Read the model definition and answer for the solid it produces. Units are mm, in the model's axes. A direction names the side the tool comes from. Coordinates: 2 decimals unless noted, no trailing zeros. Order: outer loops, then holes, each group sorted by start corner. A loop starts at its lowest first (then second) coordinate and runs counter-clockwise, first axis right, second up. Notation, with made-up numbers: M 15.5,25.25 L 57.5,25.25 A19 ccw 57.5,49.25 Z; hole C 14,-26 d8. An arc over 180 degrees is marked long. Write each question's results on one line, items separated by ' | '.
```python
from build123d import *

# Parameters (mm, degrees)
SKETCH_1_W           = 17.78
SKETCH_1_H           = 6.35
EXTRUDE_1_DEPTH      = 5.08
SKETCH_2_W           = 16.78
SKETCH_2_H           = 5.35
CUT_EXTRUDE_1_DEPTH  = 4.08
SKETCH_3_W           = 2
SKETCH_3_H           = 4.08
CUT_EXTRUDE_2_DEPTH  = 1
EXTRUDE_2_DEPTH      = 2
EXTRUDE_2_DEPTH_BACK = 3.58
SKETCH_4_W           = 0.75
SKETCH_4_H           = 0.75


with BuildPart() as part:
    # 草图1 → 拉伸1 (new body)
    with BuildSketch(Plane(origin=(0, 0, 0), x_dir=(1, 0, 0), z_dir=(0, 1, 0))):
        Rectangle(SKETCH_1_W, SKETCH_1_H)
    extrude(amount=EXTRUDE_1_DEPTH)

    # 草图2 → 切除-拉伸1 (cut)
    with BuildSketch(Plane(origin=(0, 5.08, 0), x_dir=(-1, 0, 0), z_dir=(0, 1, 0))):
        Rectangle(SKETCH_2_W, SKETCH_2_H)
    extrude(amount=-CUT_EXTRUDE_1_DEPTH, mode=Mode.SUBTRACT)

    # 草图3 → 切除-拉伸2 (cut)
    with BuildSketch(Plane.XY.offset(3.175)):
        with Locations((0, 3.04)):
            Rectangle(SKETCH_3_W, SKETCH_3_H)
    extrude(amount=-CUT_EXTRUDE_2_DEPTH, mode=Mode.SUBTRACT)

    # 草图4 → 拉伸2 (add, two sides: drawn at the far end of the back side and taken through both)
    with BuildSketch(Plane.XZ.offset(-EXTRUDE_2_DEPTH_BACK)):
        with Locations((-1.27, 0.635)):
            Rectangle(SKETCH_4_W, SKETCH_4_H)
        with Locations((1.27, 0.635)):
            Rectangle(SKETCH_4_W, SKETCH_4_H)
        with Locations((3.81, 0.635)):
            Rectangle(SKETCH_4_W, SKETCH_4_H)
        with Locations((6.35, 0.635)):
            Rectangle(SKETCH_4_W, SKETCH_4_H)
        with Locations((-3.81, 0.635)):
            Rectangle(SKETCH_4_W, SKETCH_4_H)
        with Locations((-6.35, 0.635)):
            Rectangle(SKETCH_4_W, SKETCH_4_H)
    extrude(amount=EXTRUDE_2_DEPTH + EXTRUDE_2_DEPTH_BACK)


solid = part.part
```
(1) The part is cut by section D-D, the plane y = 4.25. Write down the section's boundary in (x, z) (3 decimals), then the cut area to 3 significant figures.
Conclusion:
outline: M -8.89,-3.175 L 8.89,-3.175 L 8.89,3.175 L 1,3.175 L 1,2.675 L 8.39,2.675 L 8.39,-2.675 L -8.39,-2.675 L -8.39,2.675 L -1,2.675 L -1,3.175 L -8.89,3.175 Z | area: 22.1 mm²
(2) The part is cut by section B-B, the plane z = 1.5. Write down the section's boundary in (x, y), then the cut area to 3 significant figures.
Conclusion:
outline: M -8.89,0 L 8.89,0 L 8.89,5.08 L 8.39,5.08 L 8.39,1 L -8.39,1 L -8.39,5.08 L -8.89,5.08 Z | area: 21.9 mm²
(3) The part is cut by section A-A, the plane y = -0.75. Write down the section's boundary in (x, z) (3 decimals), then the cut area to 4 significant figures.
Conclusion:
outline: M -6.725,0.26 L -5.975,0.26 L -5.975,1.01 L -6.725,1.01 Z; M -4.185,0.26 L -3.435,0.26 L -3.435,1.01 L -4.185,1.01 Z; M -1.645,0.26 L -0.895,0.26 L -0.895,1.01 L -1.645,1.01 Z; M 0.895,0.26 L 1.645,0.26 L 1.645,1.01 L 0.895,1.01 Z; M 3.435,0.26 L 4.185,0.26 L 4.185,1.01 L 3.435,1.01 Z; M 5.975,0.26 L 6.725,0.26 L 6.725,1.01 L 5.975,1.01 Z | area: 3.375 mm²
(4) The mould has two halves that part along Z. Classify faces 3 (the flat face through (-0.1, 0.8, 3.175)), 4 (the flat face through (5, 3, 2.675)), 5 (the flat face through (0, 3, -3.175)), 6 (the flat face through (8.39, 3, 0)): pulls with the +Z half, pulls with the -Z half, needs draft (parallel to the pull), parting line crosses it, or undercut.
Conclusion:
face 3: pulls with the +Z half | face 4: undercut | face 5: pulls with the -Z half | face 6: undercut
(5) Straight lines are drawn through the part: line 1 (Z direction, x = 6.25, y = 2) (3 decimals); line 2 (X direction, y = 4.75, z = 1); line 3 (Z direction, x = 4, y = 3.75) (3 decimals). For each, find the intervals that lie inside material, in ascending order.
Conclusion:
line 1: -3.175 to -2.675, 0.26 to 1.01, 2.675 to 3.175 | line 2: -8.89 to -8.39, 8.39 to 8.89 | line 3: -3.175 to -2.675, 2.675 to 3.175
(6) Given pin 1 (0.8 mm diameter, centred on y = -1.5, z = 0.5, fed in from +X) (3 decimals); pin 2 (0.6 mm diameter, centred on x = -1.5, z = 0.5, fed in from +Y); pin 3 (0.6 mm diameter, centred on x = 6, y = -1, fed in from +Z), each flat-ended and moving along its own axis, determine where each tip first touches the part or whether it passes through.
Conclusion:
pin 1: x = 6.725 | pin 2: y = 3.58 | pin 3: z = 1.01
(7) The part is cut by section C-C, the plane x = -7.25. Write down the section's boundary in (y, z) (3 decimals).
Conclusion:
outline: M 0,-3.175 L 5.08,-3.175 L 5.08,-2.675 L 1,-2.675 L 1,2.675 L 5.08,2.675 L 5.08,3.175 L 0,3.175 Z
(8) For faces 1 (the flat face through (-1, 5.08, -3)), 2 (the flat face through (-5, 3, 2.675)), determine the directions among +Z, -Z, +X, -X, +Y, -Y from which every point of the face is accessible in a straight line to the end or side of a thin tool.
Conclusion:
face 1: +Z, -Z, +X, -X, +Y | face 2: +Y
